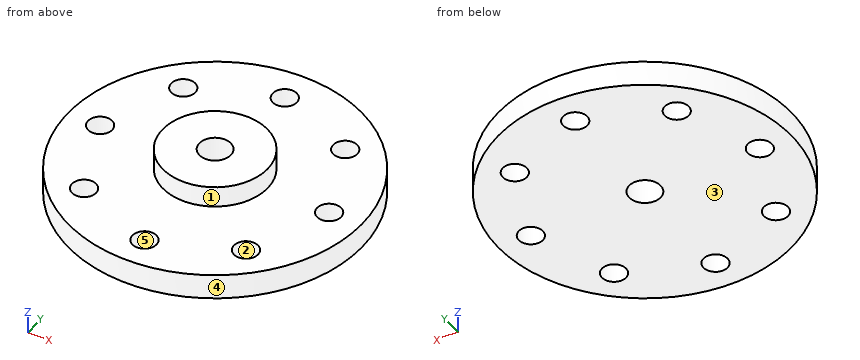
```python
from build123d import *

# Parameters (mm, degrees)
SKETCH1_R           = 14
BOSS_EXTRUDE1_DEPTH = 2.4
SKETCH2_R           = 1.15
CUT_EXTRUDE1_DEPTH  = 20.94392138
CIRPATTERN2_COUNT   = 8
SKETCH4_R           = 5
BOSS_EXTRUDE2_DEPTH = 2
SKETCH5_R           = 1.5
CUT_EXTRUDE3_DEPTH  = 21.282011735


with BuildPart() as part:
    # Sketch1 → Boss-Extrude1 (new body)
    with BuildSketch(Plane.XY):
        Circle(SKETCH1_R)
    extrude(amount=BOSS_EXTRUDE1_DEPTH)

    # Sketch2 → Cut-Extrude1 (cut, through all)
    with BuildSketch(Plane.XY.offset(2.4)):
        with Locations((0, 10.85)):
            Circle(SKETCH2_R)
    cut_extrude1 = extrude(amount=-CUT_EXTRUDE1_DEPTH, mode=Mode.SUBTRACT)

    # CirPattern2: Cut-Extrude1 ×8 about axis
    cirpattern2_axis = Axis((0, -0.073707157, 0), (0, 0, 1))
    for i in range(1, CIRPATTERN2_COUNT):
        add(cut_extrude1.rotate(cirpattern2_axis, i * 360 / CIRPATTERN2_COUNT), mode=Mode.SUBTRACT)

    # Sketch4 → Boss-Extrude2 (add)
    with BuildSketch(Plane.XY.offset(2.4)):
        Circle(SKETCH4_R)
    extrude(amount=BOSS_EXTRUDE2_DEPTH)

    # Sketch5 → Cut-Extrude3 (cut, through all)
    with BuildSketch(Plane.XY.offset(4.4)):
        Circle(SKETCH5_R)
    extrude(amount=-CUT_EXTRUDE3_DEPTH, mode=Mode.SUBTRACT)


solid = part.part
```
Could you check a few things on this model? Use its own coordinates, in mm. Face numbers are marked on the shaded views. A direction names the side the tool comes from. Round coordinates to 2 decimals unless told otherwise and drop trailing zeros. Write each loop counter-clockwise with the first axis right and the second up, starting at its lowest first coordinate (ties: lowest second). Pieces come first, ordered by that corner, then holes. Notation, with made-up numbers: M -36.75,56.25 L -24.75,56.25 A19 ccw -24.75,93.25 Z; hole C -33,82 d3. An arc over 180 degrees is marked long. Answer in a Markdown table with one row per item. Add a question column.
Q1. Imagine slicing it at D-D (y = 10.85). Please give me the cut outline in (x, z).
Q2. If we mould it in two halves opening along X, with no side actions, what happens to the marked faces 3, 4 and 5? For each: +X half, -X half, draft (parallel to the pull), parting line (faces both ways), or undercut.
Q3. On a 3-axis mill with a long thin cutter (end or side, diameter ignored), from which of +Z, -Z, +X, -X, +Y, -Y can I reach the whole of each face in a straight line? I mean the marked faces 1 and 2. Say none if no direction works.
Q4. Imagine slicing it at B-B (y = 0). Please give me the cut outline in (x, z).
Q5. Imagine slicing it at C-C (z = 1.15). Give the number of separate pieces and of enclosed holes in the cut face, then the cut area to 3 significant figures.
Q6. Imagine slicing it at A-A (x = 0). Please give me the cut outline in (y, z), then the cut area to 3 significant figures.
Q7. If I drill on line 1 (Y direction, x = 0, z = 0.6); line 2 (Y direction, x = -1, z = 1.95); line 3 (Z direction, x = 1.25, y = -8), over which ranges is the centre line in solid material (lowest first)? Write a range as from..to.
Q8. Will these pins go through, and if not, where does the flat tip stop? pin 1 Ø3 at (x, y) = (-7.72, 7.65) entering from +Z; pin 2 Ø1.4 at (x, y) = (7.72, 7.65) entering from +Z.
Values:
| question | item | result |
|---|---|---|
| 1 | outline | M -8.85,0 L -1.15,0 L -1.15,2.4 L -8.85,2.4 Z; M 1.15,0 L 8.85,0 L 8.85,2.4 L 1.15,2.4 Z |
| 2 | face 3 | draft |
| 2 | face 4 | parting line |
| 2 | face 5 | undercut |
| 3 | face 1 | +Z |
| 3 | face 2 | +Z, -Z |
| 4 | outline | M -14,0 L -12.07,0 L -12.07,2.4 L -14,2.4 Z; M -9.78,0 L -1.5,0 L -1.5,4.4 L -5,4.4 L -5,2.4 L -9.78,2.4 Z; M 1.5,0 L 9.78,0 L 9.78,2.4 L 5,2.4 L 5,4.4 L 1.5,4.4 Z; M 12.07,0 L 14,0 L 14,2.4 L 12.07,2.4 Z |
| 5 | separate pieces | 1 |
| 5 | enclosed holes | 9 |
| 5 | area | 575 mm^2 |
| 6 | outline | M -14,0 L -12.15,0 L -12.15,2.4 L -14,2.4 Z; M -9.85,0 L -1.5,0 L -1.5,4.4 L -5,4.4 L -5,2.4 L -9.85,2.4 Z; M 1.5,0 L 9.7,0 L 9.7,2.4 L 5,2.4 L 5,4.4 L 1.5,4.4 Z; M 12,0 L 14,0 L 14,2.4 L 12,2.4 Z |
| 6 | area | 63.0 mm^2 |
| 7 | line 1 | -14..-12.15, -9.85..-1.5, 1.5..9.7, 12..14 |
| 7 | line 2 | -13.96..-11.57, -10.43..-1.12, 1.12..10.28, 11.42..13.96 |
| 7 | line 3 | 0..2.4 |
| 8 | pin 1 | z = 2.4 |
| 8 | pin 2 | through |
